For this review, take the finished solid that the model builds, in its own axes (mm). Face numbers are marked on the shaded views. A direction names the side the tool comes from. Give positions to 0.01 mm unless a question says otherwise; leave off trailing zeros. Use CSV: the item, a comma, the result in double quotes. Start each with the question number.
1. Insertion check: P1, Ø1, axis at y = 4.5, z = -4, coming from the -X side; P2, Ø3, axis at x = 6.5, y = 6, coming from the -Z side; P3, Ø3, axis at y = 7.5, z = 21, coming from the -X side; P4, Ø2, axis at x = 0, z = -34.13, coming from the +Y side. Each pin has a flat end and moves straight along its axis. Give the tip position at first contact, or say it passes through.
2. Take a section at B-B, the plane x = 0. State how many separate pieces and enclosed holes the cut face has, and give its area (3 significant figures).
3. Tool access review of the marked faces 1 and 2: name each direction out of +Z, -Z, +X, -X, +Y, -Y from which nothing blocks a thin tool from reaching the whole face with its end or side.
4. To check wall thickness, follow line 1 (Y direction, x = 13.5, z = 28.5); line 2 (Y direction, x = 23, z = -21.5); line 3 (Z direction, x = 20.5, y = 11). State the ranges of each line that lie inside material, in increasing order. Write a range as [from, to].
from build123d import *

# Parameters (mm, degrees)
SKETCH1_R                       = 36.5125
EXTRUDE1_DEPTH                  = 3.175
SKETCH2_R                       = 31.75
EXTRUDE2_DEPTH                  = 9.2075
SKETCH4_W                       = 1.27
SKETCH4_H                       = 2.3622
CHAMFER1_SIZE                   = 0.381
F_2_56_TAPPED_HOLE1_D           = 1.778
F_2_56_TAPPED_HOLE1_DEPTH       = 5.588
F_2_56_TAPPED_HOLE1_CBORE_D     = 2.1844
F_2_56_TAPPED_HOLE1_CBORE_DEPTH = 4.318
F_2_56_TAPPED_HOLE1_TIP         = 0.53416509


with BuildPart() as part:
    # Sketch1 → Extrude1 (new body)
    with BuildSketch(Plane(origin=(0, 0, 0), x_dir=(1, 0, 0), z_dir=(0, 1, 0))):
        Circle(SKETCH1_R)
    extrude(amount=EXTRUDE1_DEPTH)

    # Sketch2 → Extrude2 (add)
    with BuildSketch(Plane(origin=(0, 3.175, 0), x_dir=(-1, 0, 0), z_dir=(0, 1, 0))):
        Circle(SKETCH2_R)
    extrude(amount=EXTRUDE2_DEPTH)

    # Sketch4 → Cut-Revolve7 (revolve, cut)
    with BuildSketch(Plane(origin=(0, 0, 0), x_dir=(0, 0, -1), z_dir=(1, 0, 0))):
        with Locations((-31.115, 9.224034757)):
            Rectangle(SKETCH4_W, SKETCH4_H)
        with Locations((-31.115, 5.360539726)):
            Rectangle(SKETCH4_W, SKETCH4_H)
    revolve(axis=Axis((0, 0, 0), (0, 1, 0)), mode=Mode.SUBTRACT)

    # Chamfer1
    chamfer1_edges = [part.edges().sort_by_distance(p)[0] for p in [
        (31.75, 10.405134757, 0),
        (31.75, 8.042934757, 0),
        (31.75, 6.541639726, 0),
        (31.75, 4.179439726, 0),
        (31.75, 12.3825, 0),
    ]]
    chamfer(chamfer1_edges, length=CHAMFER1_SIZE)

    # #2-56 Tapped Hole1
    with Locations(Plane(origin=(-29.558529563, 0, 17.065625), x_dir=(0, 0, -1), z_dir=(0, -1, 0))):
        with Locations((0, 0), (-17.065625, 29.558529563), (0, 59.117059126), (34.13125, 59.117059126), (51.196875, 29.558529563), (34.13125, 0)):
            CounterBoreHole(F_2_56_TAPPED_HOLE1_D / 2, F_2_56_TAPPED_HOLE1_CBORE_D / 2, F_2_56_TAPPED_HOLE1_CBORE_DEPTH, depth=F_2_56_TAPPED_HOLE1_DEPTH)
            with Locations((0, 0, -(F_2_56_TAPPED_HOLE1_DEPTH + F_2_56_TAPPED_HOLE1_TIP / 2))):  # 118° drill point
                Cone(0, F_2_56_TAPPED_HOLE1_D / 2, F_2_56_TAPPED_HOLE1_TIP, mode=Mode.SUBTRACT)


solid = part.part
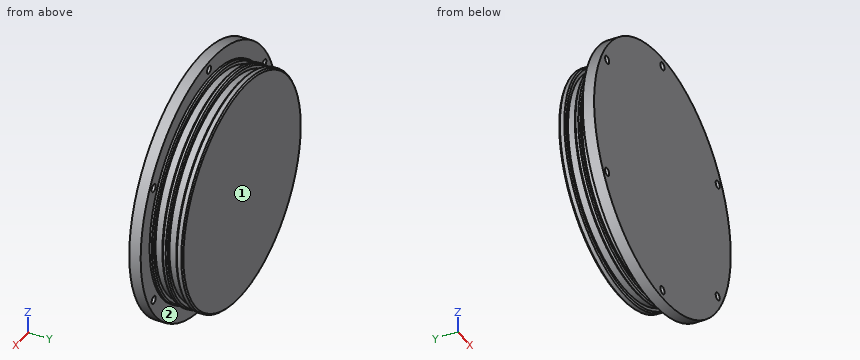
Result set:
1,P1,"x = -31.3"
1,P2,"z = -31.3"
1,P3,"x = -25.06"
1,P4,"through"
2,separate pieces,"3"
2,enclosed holes,"0"
2,area,"790 mm2"
3,face 1,"+Z, -Z, +X, -X, +Y"
3,face 2,"+Y"
4,line 1,"[0, 4.01], [6.71, 7.88], [10.57, 12.22]"
4,line 2,"[0, 4.06], [6.66, 7.93], [10.52, 12.27]"
4,line 3,"[-24.24, 24.24]"
